Here's how the part is built. I have some questions about the finished solid (model axes, mm). Round coordinates to 2 decimals unless told otherwise and drop trailing zeros. Use a Markdown table: item, result. Add a question column.
(1) If I drill on probe 1 along Y at (x, z) = (0, 2.3); probe 2 along X at (y, z) = (1.75, 0.75); probe 3 along Y at (x, z) = (-0.25, 3.7), over which ranges is the centre line in solid material (lowest first)?
(2) I'm going to push a flat-ended pin straight in: P1, Ø2, axis at x = 2.5, z = 1, coming from the -Y side. Where does the tip first touch, or does it pass through?
(3) Thinking about a two-plate mould opening in Y: for faces 1 (the face through (0, -4, 2)), 2 (the face through (-1.64, 1.26, 1.98)), 3 (the face through (1, -3, 0)), which applies, pulls with the +Y half, pulls with the -Y half, needs draft (parallel to the pull), parting line crosses it, or undercut?
Solid Edge part; units mm, degrees
sketch "Sketch1" plane through (0, 0, 0) normal (0, 0, 1) x (1, 0, 0)
  circle A0 centre (0, 0) radius 2.067
  circle A1 centre (0, 0) radius 4.6188
extrude "Protrusion1" add sketch "Sketch1" along normal blind 4
sketch "Sketch2" plane through (0, 0, 0) normal (0, 0, 1) x (1, 0, 0)
  line L0 (4.6188, 0) -> (2.3094, 4)
  arc A0 (2.3094, 4) -> (4.6188, 0) centre (0, 0) cw
extrude "ExtrudedCutout_1" cut sketch "Sketch2" along normal blind 4
pattern_circular "Pattern1" count 6 over 360 about axis through (0, 0, 0) along (0, 0, -1) of "ExtrudedCutout_1"
cosmetic_thread "Thread_1" thread depth 4
sketch "Sketch3" plane through (0, 0, 0) normal (0, -1, 0) x (1, 0, 0)
  line L0 (4.6188, 0.3645) -> (3.9875, 0)
  line L1 (3.9875, 0) -> (4.6188, 0)
  line L2 (4.6188, 0) -> (4.6188, 0.3645)
  line L3 (3.9875, 4) -> (4.6188, 4)
  line L4 (4.6188, 4) -> (4.6188, 3.6355)
  line L5 (4.6188, 3.6355) -> (3.9875, 4)
revolve "RevolvedCutout_1" cut sketch "Sketch3" angle 360 about axis through (0, 0, 8.4) along (0, 0, -1)
chamfer "Chamfer_1" distance 0.808 angle 30 1 edges at (-2.067, 0, 0) measured on face at (-2.7381, -2.5786, 0)
chamfer "Chamfer_2" distance 0.808 angle 30 1 edges at (-2.067, 0, 4) measured on face at (-2.7381, -2.5786, 4)
properties material "Stahl"
Taken from the geometry:
| question | item | result |
|---|---|---|
| 1 | probe 1 | y = -4 to -2.07, 2.07 to 4 |
| 1 | probe 2 | x = -3.61 to -1.1, 1.1 to 3.61 |
| 1 | probe 3 | y = -4 to -2.34, 2.34 to 4 |
| 2 | P1 | stops at y = -4 |
| 3 | face 1 | pulls with the -Y half |
| 3 | face 2 | undercut |
| 3 | face 3 | needs draft |
